```python
from build123d import *

# Parameters (mm, degrees)
SKETCH_1_W             = 35
SKETCH_1_H             = 25
SM_BASE_FLANGE_1_DEPTH = 5
SM_EDGE_FLANGE_1_DEPTH = 25
SM_EDGE_FLANGE_2_DEPTH = 25
CUT_EXTRUDE_1_DEPTH    = 65.707032075
CUT_EXTRUDE_3_DEPTH    = 65.707032075
SKETCH_35_R            = 4.5
CUT_EXTRUDE_2_DEPTH    = 51.227169575


# Sheet-metal steps are written as plain solids
with BuildPart() as part:
    # Sketch 1 → Базовая кромка1 (new body)
    with BuildSketch(Plane.XY):
        with Locations((0, 12.5)):
            Rectangle(SKETCH_1_W, SKETCH_1_H)
    extrude(amount=-SM_BASE_FLANGE_1_DEPTH)

    # Ребро-кромка1 section (across the edge) → Ребро-кромка1 (add)
    with BuildSketch(Plane(origin=(-20.5, 25, 0), x_dir=(1, 0, 0), z_dir=(0, -1, 0))):
        with BuildLine():
            Line((-5, 3), (-5, 31))
            Line((-5, 31), (0, 31))
            Line((0, 31), (0, 3))
            ThreePointArc((0, 3), (0.878679656, 0.878679656), (3, 0))
            Line((3, 0), (3, -5))
            ThreePointArc((3, -5), (-2.656854249, -2.656854249), (-5, 3))
        make_face()
    extrude(amount=SM_EDGE_FLANGE_1_DEPTH)

    # Ребро-кромка2 section (across the edge) → Ребро-кромка2 (add)
    with BuildSketch(Plane(origin=(20.5, 0, 0), x_dir=(-1, 0, 0), z_dir=(0, 1, 0))):
        with BuildLine():
            Line((-5, 3), (-5, 31))
            Line((-5, 31), (0, 31))
            Line((0, 31), (0, 3))
            ThreePointArc((0, 3), (0.878679656, 0.878679656), (3, 0))
            Line((3, 0), (3, -5))
            ThreePointArc((3, -5), (-2.656854249, -2.656854249), (-5, 3))
        make_face()
    extrude(amount=SM_EDGE_FLANGE_2_DEPTH)

    # Эскиз33 → Вырез-Вытянуть1 (cut, through all)
    with BuildSketch(Plane(origin=(25.5, 0, 0), x_dir=(0, 0, -1), z_dir=(1, 0, 0))):
        Polygon((-31, 0), (-31, 25), (-26.591825482, 25), align=None)
    extrude(amount=-CUT_EXTRUDE_1_DEPTH, mode=Mode.SUBTRACT)

    # Эскиз36 → Вырез-Вытянуть3 (cut, through all)
    with BuildSketch(Plane(origin=(25.5, 0, 0), x_dir=(0, 0, -1), z_dir=(1, 0, 0))):
        Polygon((-26.591825482, 25), (-27.368209794, 20.596905768), (-24.413786535, 20.075961235), (-23.545545647, 25), align=None)
        Polygon((-27.365805555, 3.334229434), (-30.320228814, 3.855173967), (-31, 0), (-27.953720164, 0), align=None)
    extrude(amount=-CUT_EXTRUDE_3_DEPTH, mode=Mode.SUBTRACT)

    # Эскиз35 → Вырез-Вытянуть2 (cut, through all)
    with BuildSketch(Plane(origin=(0, 0, -5), x_dir=(-1, 0, 0), z_dir=(0, 0, -1))):
        with Locations((0, 12.5)):
            Circle(SKETCH_35_R)
    extrude(amount=-CUT_EXTRUDE_2_DEPTH, mode=Mode.SUBTRACT)


solid = part.part
```
Part model, mm, in its own coordinate system. A direction names the side the tool comes from. Round coordinates to 2 decimals unless told otherwise and drop trailing zeros. Order: outer loops, then holes, each group sorted by start corner. A loop starts at its lowest first (then second) coordinate and runs counter-clockwise, first axis right, second up. Notation, with made-up numbers: M -21,-3 L -8,-3 A15 cw -8,21 Z; hole C 30.5,50.25 d8. An arc over 180 degrees is marked long. Answer in a Markdown table with one row per item. Add a question column.
Q1. Cut at B-B on x = 0. Give the cut face in (y, z), and give its area (3 significant figures).
Q2. Mould opens along Z. For faces 1 (the face through (23.035, 12.343, 28.824)), 2 (the face through (-22.97, 20.34, 25.91)), 3 (the face through (25.5, 12, 16)) say: +Z half, -Z half, draft (parallel to the pull), parting line (faces both ways), or undercut.
Q3. Cut at D-D on y = 18.5. Give the cut face in (x, z).
Q4. Pin check, flat tip, straight feed: pin 1 (2 mm diameter, centred on x = 5.5, y = 7.5, fed in from +Z). Stop position of the tip, or through.
Q5. Cut at A-A on z = 20.5. Give the cut face in (x, y), and give its area (3 significant figures).
Q6. Wall check: L1, parallel to X at y = 3, z = 26; L2, parallel to Y at x = 0, z = -1.4; L3, parallel to Z at x = -11, y = 20.5. Give the ranges that are in metal, low to high. Write a range as from..to.
Q7. Cut at C-C on y = 15.25. Give the cut face in (x, z).
Q8. 3-axis set-ups, long thin cutter, end or side, ignore diameter. For faces 4 (the face through (-2.419, 16.294, -2.535)), 5 (the face through (23.04, 3.59, 28.82)), 6 (the face through (-19.64, 12.68, 0.9)): which of +Z, -Z, +X, -X, +Y, -Y reach the whole face in a straight line?
Established:
| question | item | result |
|---|---|---|
| 1 | outline | M 0,-5 L 8,-5 L 8,0 L 0,0 Z; M 17,-5 L 25,-5 L 25,0 L 17,0 Z |
| 1 | area | 80.0 mm2 |
| 2 | face 1 | +Z half |
| 2 | face 2 | undercut |
| 2 | face 3 | draft |
| 3 | outline | M -25.5,3 A8 ccw -17.5,-5 L 17.5,-5 A8 ccw 25.5,3 L 25.5,27.74 L 20.5,27.74 L 20.5,3 A3 cw 17.5,0 L -17.5,0 A3 cw -20.5,3 L -20.5,27.74 L -25.5,27.74 Z |
| 4 | pin 1 | stops at z = 0 |
| 5 | outline | M -25.5,0 L -20.5,0 L -20.5,25 L -25.5,25 Z; M 20.5,0 L 25.5,0 L 25.5,25 L 20.5,25 Z |
| 5 | area | 250 mm2 |
| 6 | L1 | x = -25.5..-20.5, 20.5..25.5 |
| 6 | L2 | y = 0..8, 17..25 |
| 6 | L3 | z = -5..0 |
| 7 | outline | M -25.5,3 A8 ccw -17.5,-5 L -3.56,-5 L -3.56,0 L -17.5,0 A3 cw -20.5,3 L -20.5,28.31 L -25.5,28.31 Z; M 3.56,-5 L 17.5,-5 A8 ccw 25.5,3 L 25.5,28.31 L 20.5,28.31 L 20.5,3 A3 cw 17.5,0 L 3.56,0 Z |
| 8 | face 4 | +Z, -Z |
| 8 | face 5 | +Z, +X, -X |
| 8 | face 6 | +Z, +Y, -Y |
